from build123d import *

# Parameters (mm, degrees)
F0_W     = 25.4
F0_H     = 25.4
F0_R     = 7.9375
F0_R_2   = 5.8024107256
F1_DEPTH = 38.1
F2_DEPTH = 127
F4_START = -12.7
F3_R     = 2.4554456834
F4_DEPTH = 63.5


with BuildPart() as f1:
    # F0 (on Front) → F1 (new body)
    with BuildSketch(Plane.XZ):
        Rectangle(F0_W, F0_H)
        Circle(F0_R, mode=Mode.SUBTRACT)
        Circle(F0_R)
        Circle(F0_R_2, mode=Mode.SUBTRACT)
    extrude(amount=F1_DEPTH)

    # F0 (on Front) → F2 (join)
    with BuildSketch(Plane.XZ):
        Circle(F0_R)
        Circle(F0_R_2, mode=Mode.SUBTRACT)
    extrude(amount=F2_DEPTH)

    # F3 (on face) → F4 (cut)
    with BuildSketch(Plane.XZ.offset(127).offset(F4_START)):
        with Locations((9.5774363726, 0)):
            Circle(F3_R)
        with Locations((5.9714339063, 7.4879412775)):
            Circle(F3_R)
        with Locations((-2.1311800865, 9.3373100468)):
            Circle(F3_R)
        with Locations((-8.6289720061, 4.1554939045)):
            Circle(F3_R)
        with Locations((-8.6289720061, -4.1554939045)):
            Circle(F3_R)
        with Locations((-2.1311800865, -9.3373100468)):
            Circle(F3_R)
        with Locations((5.9714339063, -7.4879412775)):
            Circle(F3_R)
    extrude(amount=-F4_DEPTH, mode=Mode.SUBTRACT)


solid = f1.part
Check sheet for the modelled part. Datum: model origin and axes. Units: mm. A direction names the side the tool comes from. Give positions to 0.01 mm unless a question says otherwise; leave off trailing zeros. Loops run counter-clockwise (first coordinate to the right, second up) from the corner with the lowest first, then second, coordinate; pieces in that order, holes last. Notation, with made-up numbers: M 11,-23.75 L 51,-23.75 A22 cw 51,2.25 Z; hole C -36.5,48 d8. An arc over 180 degrees is marked long. Return JSON: item names as keys, results as strings. Group by question number.
1. Tool access check on faces 1 (the cylindrical face through (-1.61, -82.994, 6.938)), 2 (the flat face through (-6, -38.1, 6)), 3 (the cylindrical face through (7.122, -82.994, 0.025)), 4 (the cylindrical face through (-6.428, -82.994, 3.067)). Record the directions out of +Z, -Z, +X, -X, +Y, -Y that give a thin tool (end or side, any length) a straight path to the whole face; none if there is none.
2. Cross-section at C-C on z = 10.75. Record the boundary of the cut face in (x, y), plus the area to 3 significant figures.
3. Cross-section at D-D on y = -42. Record the boundary of the cut face in (x, z) (1 decimal), plus the area to 3 significant figures.
4. Cross-section at B-B on y = -22.5. Record the boundary of the cut face in (x, z).
5. Cross-section at A-A on z = 0. Record the boundary of the cut face in (x, y).
6. Thickness scan on L1, parallel to X at y = -43.5, z = -0.25; L2, parallel to Z at x = 0.5, y = -5; L3, parallel to Z at x = 0, y = -68.5. Record the ranges inside material, lowest first.
7. Go/stop test with flat-tipped pins: pin 1 (1 mm diameter, centred on x = -6.5, y = -50, fed in from -Z); pin 2 (1.5 mm diameter, centred on y = -41.5, z = 8, fed in from -X); pin 3 (4 mm diameter, centred on x = 0, y = -69.5, fed in from +Z). Record where each tip stops, or that it passes through.
8. Mould release check, pull along X, two halves, no side actions. Record for faces 5 (the cylindrical face through (-5.85, -81.928, 5.365)), 6 (the cylindrical face through (5.534, -62.611, 1.743)), 7 (the flat face through (12.7, -19, 0)), 8 (the flat face through (0, -19, -12.7)): released by +X, released by -X, zero draft, split by the parting line, or undercut.
Return value:
{
 "1": {"face 1": "+Z", "face 2": "-Y", "face 3": "+X", "face 4": "-X"},
 "2": {"outline": "M -12.7,-38.1 L 12.7,-38.1 L 12.7,0 L -12.7,0 Z", "area": "968 mm^2"},
 "3": {"outline": "C 0,0 d15.9; hole C 0,0 d11.6", "area": "92.2 mm^2"},
 "4": {"outline": "M -12.7,-12.7 L 12.7,-12.7 L 12.7,12.7 L -12.7,12.7 Z; hole C 0,0 d11.6"},
 "5": {"outline": "M -12.7,-38.1 L -7.94,-38.1 L -7.94,-127 L -5.8,-127 L -5.8,0 L -12.7,0 Z; M 5.8,-127 L 7.94,-127 L 7.94,-114.3 L 7.12,-114.3 L 7.12,-50.8 L 7.94,-50.8 L 7.94,-38.1 L 12.7,-38.1 L 12.7,0 L 5.8,0 Z"},
 "6": {"L1": "-7.93 to -5.8, 5.8 to 7.93", "L2": "-12.7 to -5.78, 5.78 to 12.7", "L3": "-7.94 to -5.8, 5.8 to 7.94"},
 "7": {"pin 1": "z = -5.2", "pin 2": "x = -3.23", "pin 3": "z = 7.94"},
 "8": {"face 5": "split by the parting line", "face 6": "undercut", "face 7": "released by +X", "face 8": "zero draft"}
}
